Autodesk Inventor part; units mm, degrees
ref_plane "YZ Plane" through (0, 0, 0) normal (1, 0, 0) x (0, 1, 0)
ref_plane "XZ Plane" through (0, 0, 0) normal (0, 1, 0) x (-1, 0, 0)
ref_plane "XY Plane" through (0, 0, 0) normal (0, 0, 1) x (1, 0, 0)
sketch "Sketch1" plane through (0, 0, 0) normal (0, 1, 0) x (-1, 0, 0)
  line L0 (74.75, 74.575) -> (-74.75, 74.575)
  line L1 (-74.75, 74.575) -> (-74.75, -74.575)
  line L2 (-74.75, -74.575) -> (74.75, -74.575)
  line L3 (74.75, -74.575) -> (74.75, 74.575)
  line L4 (74.75, 74.575) -> (-74.75, -74.575) construction
  line L5 (-74.75, 74.575) -> (74.75, -74.575) construction
  point P0 (0, 0)
  dimension "d32" = 149.5
  dimension "d33" = 149.15
extrude "Extrusion1" add sketch "Sketch1" against normal blind 4.064
hole "Hole4" at (60, 0, -60) direction (0, -1, 0) diameter 4.5 depth 4.064 countersink diameter 9.4 countersink angle 90
hole "Hole3" at (-60, 0, 60) direction (0, -1, 0) diameter 4.5 depth 4.064 countersink diameter 9.4 countersink angle 90
sketch "Sketch3" plane through (0, 0, 0) normal (0, 1, 0) x (-1, 0, 0)
  point P0 (60, 60)
hole "Hole2" at (60, 0, 60) direction (0, -1, 0) diameter 4.5 depth 4.064 countersink diameter 9.4 countersink angle 90
sketch "Sketch2" plane through (0, 0, 0) normal (0, 1, 0) x (-1, 0, 0)
  point P0 (-60, -60)
hole "Hole1" at (-60, 0, -60) direction (0, -1, 0) diameter 4.5 depth 4.064 countersink diameter 9.4 countersink angle 90
sketch "Sketch4" plane through (0, 0, 0) normal (0, 1, 0) x (-1, 0, 0)
  point P0 (-60, 60)
sketch "Sketch5" plane through (0, 0, 0) normal (0, 1, 0) x (-1, 0, 0)
  point P0 (60, -60)
properties part number "Piston Build surface" material "Aluminum 6061"
For this review, take the finished solid that the model builds, in its own axes (mm). Give positions to 0.01 mm unless a question says otherwise; leave off trailing zeros. Write each loop counter-clockwise with the first axis right and the second up, starting at its lowest first coordinate (ties: lowest second). Pieces come first, ordered by that corner, then holes.
Item 1: Wall thickness on probe 1 along Z at (x, y) = (60, -2.95) (3 decimals); probe 2 along X at (y, z) = (-2.9, 60); probe 3 along Z at (x, y) = (61.5, -3.55) (3 decimals): over which ranges is each line inside the solid? List them lowest first.
Item 2: The part is to be moulded in two halves that separate along X. For faces 1 (the face through (74.75, -2, 1)), 2 (the face through (1, -2, -74.575)), 3 (the face through (59.08, -2.297, -57.78)), 4 (the face through (-60.92, -2.297, 62.22)), say which applies: +X half, -X half, draft (parallel to the pull), parting line (faces both ways), or undercut.
Item 3: Take a section at A-A (x = -60). Give the boundary of the cut face in (y, z) (3 decimals), and give its area (3 significant figures).
Item 4: Insertion check: P1, Ø7, axis at x = -60, z = 60, coming from the +Y side. The pin has a flat end and moves straight along its axis. Give the tip position at first contact, or say it passes through.
Item 5: Take a section at B-B (z = 60). Give the boundary of the cut face in (x, y).
Established:
1. probe 1: z = -74.575 to -62.25, -57.75 to 57.75, 62.25 to 74.575
1. probe 2: x = -74.75 to -62.25, -57.75 to 57.75, 62.25 to 74.75
1. probe 3: z = -74.575 to -61.677, -58.323 to 58.323, 61.677 to 74.575
2. face 1: +X half
2. face 2: draft
2. face 3: undercut
2. face 4: undercut
3. outline: (-4.064, -74.575) - (0, -74.575) - (0, -64.7) - (-2.45, -62.25) - (-4.064, -62.25) - close; (-4.064, -57.75) - (-2.45, -57.75) - (0, -55.3) - (0, 55.3) - (-2.45, 57.75) - (-4.064, 57.75) - close; (-4.064, 62.25) - (-2.45, 62.25) - (0, 64.7) - (0, 74.575) - (-4.064, 74.575) - close
3. area: 558 mm2
4. P1: stops at y = -1.2
5. outline: (-74.75, -4.06) - (-62.25, -4.06) - (-62.25, -2.45) - (-64.7, 0) - (-74.75, 0) - close; (-57.75, -4.06) - (57.75, -4.06) - (57.75, -2.45) - (55.3, 0) - (-55.3, 0) - (-57.75, -2.45) - close; (62.25, -4.06) - (74.75, -4.06) - (74.75, 0) - (64.7, 0) - (62.25, -2.45) - close
